Read the model definition and answer for the solid it produces. Units are mm, in the model's axes. A direction names the side the tool comes from. Give positions to 0.01 mm unless a question says otherwise; leave off trailing zeros. Loops run counter-clockwise (first coordinate to the right, second up) from the corner with the lowest first, then second, coordinate; pieces in that order, holes last.
(1) Find section B-B, the plane y = 5. Write down the section's boundary in (x, z) (3 decimals), then the cut area to 3 significant figures.
(2) Straight lines are drawn through the part: probe 1 along Y at (x, z) = (3, 231); probe 2 along X at (y, z) = (-51, 252.5) (3 decimals); probe 3 along X at (y, z) = (-36, 225) (3 decimals). For each, find the intervals that lie inside material, in ascending order.
(3) Each of these flat-tipped pins is pushed along its axis until it touches: P1, Ø4, axis at x = -7.5, z = 259, coming from the +Y side; P2, Ø24, axis at y = -14, z = 250, coming from the +X side (3 decimals); P3, Ø1.1, axis at x = -21.5, y = 81.5, coming from the -Z side. Where does it stop, or does it pass through?
(4) Find section C-C, the plane x = -6.5. Write down the section's boundary in (y, z) (3 decimals), then the cut area to 3 significant figures.
(5) Find section A-A, the plane z = 227. Write down the section's boundary in (x, y) (3 decimals), then the cut area to 3 significant figures.
(6) Which of the six approach directions +Z, -Z, +X, -X, +Y, -Y give full straight-line access (tool end or side, diameter ignored) to faces 4 (the face through (1, -97.663, 237)), 5 (the face through (-1, 86.36, 245)), 6 (the face through (-1, 80.899, 258))?
(7) Determine the mould class of faces 1 (the face through (-57, 13, 230.2)), 2 (the face through (-47.625, -8, 239)), 3 (the face through (-53.975, -8, 245)) for opening direction X: pulls with the +X half, pulls with the -X half, needs draft (parallel to the pull), parting line crosses it, or undercut.
(8) Find section D-D, the plane z = 246. Write down the section's boundary in (x, y) (3 decimals), then the cut area to 3 significant figures.
```python
from build123d import *

# Parameters (mm, degrees)
SKETCH1_W           = 127
SKETCH1_H           = 196.088
EXTRUDE1_DEPTH      = 230.2002
SKETCH5_W           = 107.95
SKETCH5_H           = 186.563
EXTRUDE4_DEPTH      = 30.15234
EXTRUDE2_DEPTH      = 93.98
EXTRUDE2_DEPTH_BACK = 273.8502
SKETCH4_W           = 95.25
SKETCH4_H           = 132.588
SKETCH6_W           = 95.25
SKETCH6_H           = 45.974
SKETCH6_H_2         = 2.921
EXTRUDE5_DEPTH      = 256.54
FILLET1_R           = 2.54
SKETCH2_R           = 222.758
EXTRUDE3_DEPTH      = 202.86
FILLET2_R           = 0.635


with BuildPart() as part:
    # Sketch1 → Extrude1 (new body)
    with BuildSketch(Plane.XY):
        with Locations((0, -2.159)):
            Rectangle(SKETCH1_W, SKETCH1_H)
    extrude(amount=EXTRUDE1_DEPTH)

    # Sketch5 → Extrude4 (add)
    with BuildSketch(Plane.XY.offset(230.2002)):
        with Locations((0, -6.9215)):
            Rectangle(SKETCH5_W, SKETCH5_H)
    extrude(amount=EXTRUDE4_DEPTH)

    # Sketch4 → Extrude2 (cut, two sides: drawn at the far end of the back side and taken through both)
    with BuildSketch(Plane.XY.offset(230.2002).offset(-EXTRUDE2_DEPTH_BACK)):
        with Locations((0, 14.605)):
            Rectangle(SKETCH4_W, SKETCH4_H)
    extrude(amount=EXTRUDE2_DEPTH + EXTRUDE2_DEPTH_BACK, mode=Mode.SUBTRACT)

    # Sketch6 → Extrude5 (cut)
    with BuildSketch(Plane(origin=(0, 0, 0), x_dir=(-1, 0, 0), z_dir=(0, 0, -1))):
        with Locations((0, -74.676)):
            Rectangle(SKETCH6_W, SKETCH6_H)
        with Locations((0, 82.3595)):
            Rectangle(SKETCH6_W, SKETCH6_H_2)
    extrude(amount=-EXTRUDE5_DEPTH, mode=Mode.SUBTRACT)

    # Fillet1
    fillet1_edges = [part.edges().sort_by_distance(p)[0] for p in [
        (47.625, -97.663, 128.27),
        (-47.625, -97.663, 128.27),
        (47.625, 83.82, 128.27),
        (-47.625, 83.82, 128.27),
    ]]
    fillet(fillet1_edges, radius=FILLET1_R)

    # Sketch2 → Extrude3 (cut)
    with BuildSketch(Plane(origin=(0, 95.885, 0), x_dir=(-1, 0, 0), z_dir=(0, 1, 0))):
        Circle(SKETCH2_R)
    extrude(amount=-EXTRUDE3_DEPTH, mode=Mode.SUBTRACT)

    # Fillet2
    fillet2_edges = [part.edges().sort_by_distance(p)[0] for p in [
        (-47.625, 80.899, 258.44627),
        (-47.625, -51.689, 258.44627),
        (47.625, -51.689, 258.44627),
        (47.625, 80.899, 258.44627),
    ]]
    fillet(fillet2_edges, radius=FILLET2_R)


solid = part.part
```
Entries:
1. outline: (-63.5, 213.516) arc R222.758 cw to (-47.625, 217.607) - (-47.625, 260.353) - (-53.975, 260.353) - (-53.975, 230.2) - (-63.5, 230.2) - close; (47.625, 217.607) arc R222.758 cw to (63.5, 213.516) - (63.5, 230.2) - (53.975, 230.2) - (53.975, 260.353) - (47.625, 260.353) - close
1. area: 844 mm2
2. probe 1: y = -100.2 to -97.66, 83.82 to 86.36
2. probe 2: x = -53.975 to -47.625, 47.625 to 53.975
2. probe 3: x = -63.5 to -47.625, 47.625 to 63.5
3. P1: stops at y = 86.36
3. P2: stops at x = 53.975
3. P3: stops at z = 256.54
4. outline: (-100.203, 222.663) - (-97.663, 222.663) - (-97.663, 256.54) - (-51.689, 256.54) - (-51.689, 260.353) - (-100.203, 260.353) - close; (80.899, 256.54) - (83.82, 256.54) - (83.82, 222.663) - (95.885, 222.663) - (95.885, 230.2) - (86.36, 230.2) - (86.36, 260.353) - (80.899, 260.353) - close
4. area: 450 mm2
5. outline: (-63.5, -100.203) - (63.5, -100.203) - (63.5, 95.885) - (-63.5, 95.885) - close; hole (-47.625, -95.123) arc R2.54 ccw to (-45.085, -97.663) - (45.085, -97.663) arc R2.54 ccw to (47.625, -95.123) - (47.625, 81.28) arc R2.54 ccw to (45.085, 83.82) - (-45.085, 83.82) arc R2.54 ccw to (-47.625, 81.28) - close
5. area: 7,620 mm2
6. face 4: -Z
6. face 5: +Z, +X, -X, +Y
6. face 6: +Z, -Z
7. face 1: needs draft
7. face 2: undercut
7. face 3: pulls with the -X half
8. outline: (-53.975, -100.203) - (53.975, -100.203) - (53.975, 86.36) - (-53.975, 86.36) - close; hole (-47.625, -95.123) arc R2.54 ccw to (-45.085, -97.663) - (45.085, -97.663) arc R2.54 ccw to (47.625, -95.123) - (47.625, 81.28) arc R2.54 ccw to (45.085, 83.82) - (-45.085, 83.82) arc R2.54 ccw to (-47.625, 81.28) - close
8. area: 2,860 mm2
